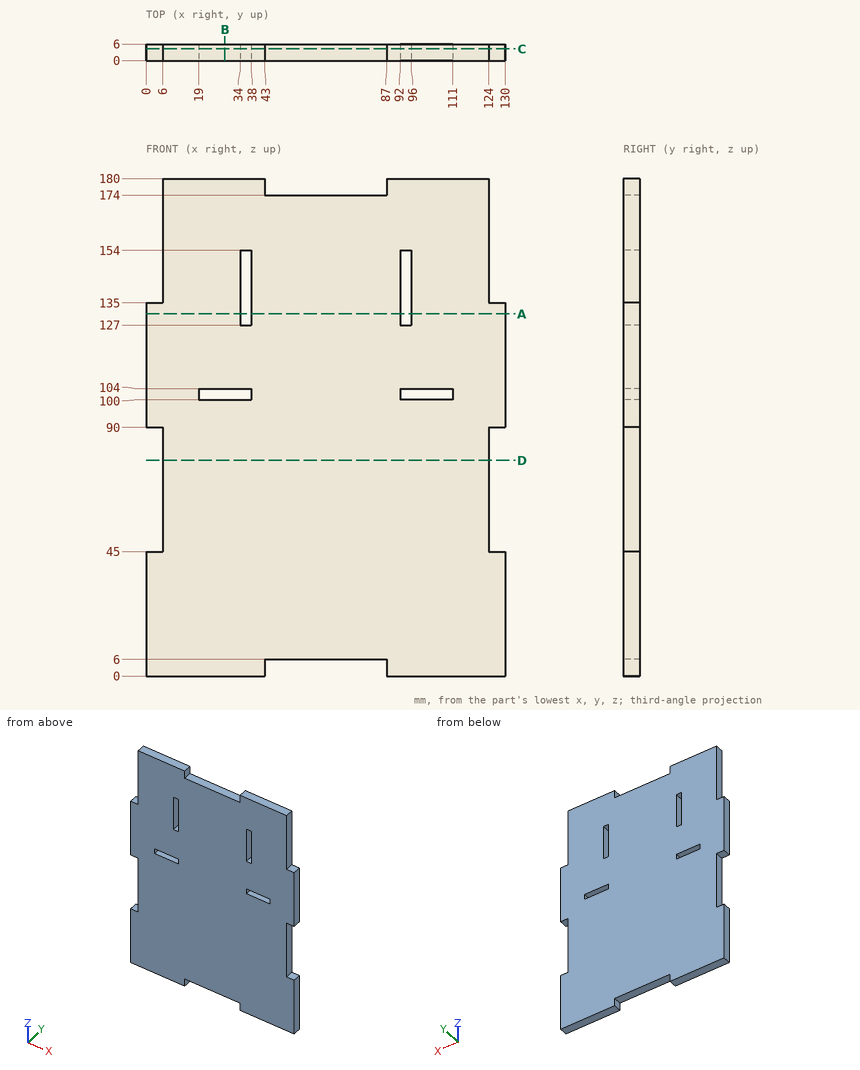
Source: three-view drawing plus pictorial views. Frame: mm from the lowest corner of the part. Coordinates: 2 decimals unless noted, no trailing zeros. Order: outer loops, then holes, each group sorted by start corner. A loop starts at its lowest first (then second) coordinate and runs counter-clockwise, first axis right, second up. Notation, with made-up numbers: M 12.25,2.25 L 48.25,2.25 A18 ccw 48.25,24.25 Z; hole C 67.25,-30.75 d8. An arc over 180 degrees is marked long. Answer in a Markdown table with one row per item.
(1) Material intervals for line 1 (X direction, y = 2.4, z = 153.5); line 2 (Z direction, x = 124.5, y = 4.15); line 3 (Z direction, x = 22.5, y = 4.25), sorted ascending. Write a range as [from, to].
Numbers:
| item | result |
|---|---|
| line 1 | x = [6, 34], [38, 92], [96, 124] |
| line 2 | z = [0, 45], [90, 135] |
| line 3 | z = [0, 100], [104, 180] |
(2) Section query D-D, the plane z = 78. Output: boundary loops of the cut face in (x, y), plus the area to 3 significant figures.
Numbers:
| item | result |
|---|---|
| outline | M 6,0 L 124,0 L 124,6 L 6,6 Z |
| area | 708 mm^2 |
(3) Section query C-C, the plane y = 4.25. Give the number of separate pieces and of enclosed holes in the cut face, plus the area to 3 significant figures.
Numbers:
| item | result |
|---|---|
| separate pieces | 1 |
| enclosed holes | 4 |
| area | 21,400 mm^2 |
(4) Section query B-B, the plane x = 28.5. Output: boundary loops of the cut face in (y, z).
Numbers:
| item | result |
|---|---|
| outline | M 0,0 L 6,0 L 6,100 L 0,100 Z; M 0,104 L 6,104 L 6,180 L 0,180 Z |
(5) Section query A-A, the plane z = 131. Output: boundary loops of the cut face in (x, y).
Numbers:
| item | result |
|---|---|
| outline | M 0,0 L 34,0 L 34,6 L 0,6 Z; M 38,0 L 92,0 L 92,6 L 38,6 Z; M 96,0 L 130,0 L 130,6 L 96,6 Z |
(6) Contact query for flat-ended pins moving along their axis: pin 1 Ø3 at (x, y) = (60.5, 4.5) entering from +Z; pin 2 Ø1.5 at (x, y) = (52.5, 3.5) entering from -Z; pin 3 Ø3 at (y, z) = (4, 177.5) entering from +X. Output: stop coordinate, or through.
Numbers:
| item | result |
|---|---|
| pin 1 | stops at z = 174 |
| pin 2 | stops at z = 6 |
| pin 3 | stops at x = 124 |
